from build123d import *

# Parameters (mm, degrees)
SKETCH1_W                  = 180
SKETCH1_H                  = 350
BOSS_EXTRUDE1_DEPTH        = 4
F_22_0_22_DIAMETER_HOLE1_D = 22
LPATTERN1_COUNT            = 5
LPATTERN1_PITCH            = 70


with BuildPart() as part:
    # Sketch1 → Boss-Extrude1 (new, symmetric)
    with BuildSketch(Plane.XY):
        Rectangle(SKETCH1_W, SKETCH1_H)
    extrude(amount=BOSS_EXTRUDE1_DEPTH, both=True)

    # Ø22.0 (22) Diameter Hole1 (through all)
    with Locations(Plane.XY.offset(4)):
        with Locations((-60, 140), (60, 140)):
            f_22_0_22_diameter_hole1 = Hole(F_22_0_22_DIAMETER_HOLE1_D / 2)

    # LPattern1: Ø22.0 (22) Diameter Hole1 ×5
    with Locations(*[(0, -i * LPATTERN1_PITCH, 0) for i in range(1, LPATTERN1_COUNT)]):
        add(f_22_0_22_diameter_hole1, mode=Mode.SUBTRACT)


solid = part.part
Geometry: final body of the model. Coordinates: model frame, mm. Round coordinates to 2 decimals unless told otherwise and drop trailing zeros. Order: outer loops, then holes, each group sorted by start corner. A loop starts at its lowest first (then second) coordinate and runs counter-clockwise, first axis right, second up. Notation, with made-up numbers: (73, 35.25) -> (81, 35.25) arc R15 ccw to (81, 49.25) -> close; hole circle Ø6 at (82.25, 86.25). An arc over 180 degrees is marked (long way). Put each result on its own line as item: value. Start each with the question number.
Q1. Section B-B on z = -1. Give the number of separate pieces and of enclosed holes in the cut face, and give its area (3 significant figures).
Q2. Section A-A on y = 70. Return the cut outline in (x, z).
Q3. Pull-direction query (Y, two-part tool) for faces 1 (the flat face through (-1, 175, 0)), 2 (the cylindrical face through (71, 70, 0)), 3 (the flat face through (-90, -2, 0)), 4 (the cylindrical face through (-58.568, -129.094, -0.056)); classes: +Y half, -Y half, draft (parallel to the pull), parting line (faces both ways), or undercut.
Q4. Line query: probe 1 along Y at (x, z) = (60, 0.5); probe 2 along X at (y, z) = (-144, 1); probe 3 along Y at (x, z) = (-64, 1.25). Output: solid intervals per line, ascending.
Ans:
1. separate pieces: 1
1. enclosed holes: 10
1. area: 59,200 mm2
2. outline: (-90, -4) -> (-71, -4) -> (-71, 4) -> (-90, 4) -> close; (-49, -4) -> (49, -4) -> (49, 4) -> (-49, 4) -> close; (71, -4) -> (90, -4) -> (90, 4) -> (71, 4) -> close
3. face 1: +Y half
3. face 2: undercut
3. face 3: draft
3. face 4: undercut
4. probe 1: y = -175 to -151, -129 to -81, -59 to -11, 11 to 59, 81 to 129, 151 to 175
4. probe 2: x = -90 to -70.25, -49.75 to 49.75, 70.25 to 90
4. probe 3: y = -175 to -150.25, -129.75 to -80.25, -59.75 to -10.25, 10.25 to 59.75, 80.25 to 129.75, 150.25 to 175
